Source: CAD feature listing. Evaluate the final solid. Frame: model axes, mm. A direction names the side the tool comes from. Give positions to 0.01 mm unless a question says otherwise; leave off trailing zeros. Write each loop counter-clockwise with the first axis right and the second up, starting at its lowest first coordinate (ties: lowest second). Pieces come first, ordered by that corner, then holes. Notation, with made-up numbers: (58.25, 71) - (64.25, 71) arc R27 ccw to (64.25, 89) - close; hole circle Ø7 at (49.5, 87.5). An arc over 180 degrees is marked (long way). Answer as a JSON object with one key per item and string values. Group by question number.
Autodesk Inventor part; units mm, degrees
ref_plane "YZ Plane" through (0, 0, 0) normal (1, 0, 0) x (0, 1, 0)
ref_plane "XZ Plane" through (0, 0, 0) normal (0, 1, 0) x (-1, 0, 0)
ref_plane "XY Plane" through (0, 0, 0) normal (0, 0, 1) x (1, 0, 0)
sketch "Sketch1" plane through (0, 0, 0) normal (0, 0, 1) x (1, 0, 0)
  line L0 (0, 0) -> (-75, 0)
  line L1 (-75, 0) -> (-75, 180)
  line L2 (-75, 180) -> (0, 180)
  line L3 (0, 180) -> (0, 0)
  line L4 (-65, 170) -> (-10, 170)
  line L5 (-10, 10) -> (-65, 10)
  line L6 (-65, 10) -> (-65, 85)
  line L7 (-65, 95) -> (-65, 170)
  line L8 (-10, 170) -> (-10, 95)
  line L9 (-10, 85) -> (-10, 10)
  line L10 (-65, 85) -> (-65, 95)
  line L11 (-10, 95) -> (-10, 85)
  point P0 (-65, 90)
  point P1 (-10, 90)
  dimension "d35" = 75
  dimension "d36" = 180
  dimension "d37" = 55
  dimension "d38" = 160
extrude "Extrusion7" add sketch "Sketch1" along normal blind 70
sketch "Sketch4" plane through (0, 0, 70) normal (0, 0, 1) x (1, 0, 0)
  line L0 (-75, 0) -> (0, 0)
  line L1 (0, 180) -> (-75, 180)
  line L2 (0, 0) -> (-75, 0)
  line L3 (-75, 0) -> (-75, 180)
  line L4 (-75, 180) -> (0, 180)
  line L5 (0, 180) -> (0, 0)
extrude "Extrusion8" add sketch "Sketch4" along normal blind 5
sketch "Sketch5" plane through (0, 0, 75) normal (0, 0, 1) x (1, 0, 0)
  line L0 (-65, 85) -> (-65, 95)
  line L1 (-10, 95) -> (-10, 85)
  line L2 (-10, 62.5) -> (-10, 90)
  line L3 (-10, 62.5) -> (-65, 62.5)
  line L4 (-65, 62.5) -> (-65, 117.5)
  line L5 (-65, 117.5) -> (-10, 117.5)
  line L6 (-10, 117.5) -> (-10, 62.5)
  point P0 (-65, 90)
  dimension "d59" = 55
  dimension "d60" = 55
extrude "Extrusion9" cut sketch "Sketch5" against normal blind 2
sketch "Sketch6" plane through (0, 0, 0) normal (1, 0, 0) x (0, 0, -1)
  line L0 (-10, 62.5) -> (-65, 62.5)
  line L1 (-65, 62.5) -> (-65, 117.5)
  line L2 (-65, 117.5) -> (-10, 117.5)
  line L3 (-10, 117.5) -> (-10, 62.5)
  dimension "d67" = 55
  dimension "d68" = 55
extrude "Extrusion10" cut sketch "Sketch6" against normal blind 2
sketch "Sketch7" plane through (-75, 0, 0) normal (-1, 0, 0) x (0, 0, 1)
  line L0 (10, 62.5) -> (65, 62.5)
  line L1 (10, 62.5) -> (65, 62.5)
  line L2 (65, 62.5) -> (65, 117.5)
  line L3 (65, 117.5) -> (10, 117.5)
  line L4 (10, 117.5) -> (10, 62.5)
  point P0 (0, 0)
  dimension "d71" = 55
  dimension "d72" = 55
extrude "Extrusion11" cut sketch "Sketch7" against normal blind 2
sketch "Sketch8" plane through (-75, 0, 0) normal (0, -1, 0) x (1, 0, 0)
  line L0 (10, 10) -> (65, 10)
  line L1 (65, 10) -> (65, 65)
  line L2 (65, 65) -> (10, 65)
  line L3 (10, 65) -> (10, 10)
  point P0 (75, 0)
  dimension "d75" = 55
  dimension "d76" = 55
extrude "Extrusion12" cut sketch "Sketch8" against normal blind 2
sketch "Sketch9" plane through (-75, 180, 0) normal (0, 1, 0) x (1, 0, 0)
  line L0 (10, -10) -> (65, -10)
  line L1 (65, -10) -> (65, -65)
  line L2 (65, -65) -> (10, -65)
  line L3 (10, -65) -> (10, -10)
  point P0 (75, 0)
  dimension "d79" = 55
  dimension "d80" = 55
extrude "Extrusion13" cut sketch "Sketch9" against normal blind 2
sketch "Sketch10" plane through (-75, 0, 0) normal (0, -1, 0) x (1, 0, 0)
  line L0 (74, 1) -> (63.4, 1)
  line L1 (63.4, 1) -> (63.4, 6.6)
  line L2 (63.4, 6.6) -> (74, 6.6)
  line L3 (74, 6.6) -> (74, 1)
  line L4 (1, 1) -> (11.6, 1)
  line L5 (11.6, 1) -> (11.6, 6.6)
  line L6 (11.6, 6.6) -> (1, 6.6)
  line L7 (1, 6.6) -> (1, 1)
  point P0 (75, 0)
  dimension "d83" = 10.6
  dimension "d84" = 5.6
  dimension "d85" = 10.6
  dimension "d86" = 5.6
extrude "Extrusion14" cut sketch "Sketch10" against normal blind 5
sketch "Sketch11" plane through (-75, 180, 0) normal (0, 1, 0) x (1, 0, 0)
  line L0 (1, -1) -> (11.6, -1)
  line L1 (11.6, -1) -> (11.6, -6.6)
  line L2 (11.6, -6.6) -> (1, -6.6)
  line L3 (1, -6.6) -> (1, -1)
  line L4 (74, -1) -> (63.4, -1)
  line L5 (63.4, -1) -> (63.4, -6.6)
  line L6 (63.4, -6.6) -> (74, -6.6)
  line L7 (74, -6.6) -> (74, -1)
  point P0 (75, 0)
  dimension "d89" = 10.6
  dimension "d90" = 5.6
  dimension "d91" = 10.6
  dimension "d92" = 5.6
extrude "Extrusion15" cut sketch "Sketch11" against normal blind 5
properties part number "Shoulder_Cube_TestFit_V1"
Q1. Draft query along X for faces 5 (the flat face through (0, 91, 4)), 6 (the flat face through (-75, 89, 4)), 7 (the flat face through (-38, 180, 70)), 8 (the flat face through (-69, 178, 1)). Return one class per face: released by +X, released by -X, zero draft, split by the parting line, or undercut.
Q2. First-contact query: pin 1 Ø1.5 at (x, z) = (-25.5, 39.5) entering from +Y; pin 2 Ø2 at (x, z) = (-45, 34.5) entering from -Y; pin 3 Ø12 at (y, z) = (110, 55.5) entering from -X. Flat tips, straight axial feed; report the tip coordinate or a pass-through.
Q3. Section A-A on z = 53. Return the cut outline in (x, y), then the cut area to 3 significant figures.
Q4. Ray query, probe 1 along X at (y, z) = (72.5, 26.5); probe 2 along X at (y, z) = (75, 8); probe 3 along Y at (x, z) = (-19.5, 31.5). Return the intervals inside material, ascending. Write a range as [from, to].
Q5. Reachability of faces 1 (the flat face through (-5, 91, 75)), 2 (the flat face through (-69, 2, 6.6)), 3 (the flat face through (-69, 175, 4)), 4 (the flat face through (-38, 91, 70)) from +Z, -Z, +X, -X, +Y, -Y: full face, straight path, thin tool, end or side. Return the list, or none.
Q6. Section C-C on x = -49.5. Return the cut outline in (y, z).
Q7. Section D-D on y = 106. Return the cut outline in (x, z), then the cut area to 4 significant figures.
Q8. Section B-B on y = 132.5. Return the cut outline in (x, z), then the cut area to 4 significant figures.
Taken from the geometry:
{
 "1": {"face 5": "released by +X", "face 6": "released by -X", "face 7": "zero draft", "face 8": "undercut"},
 "2": {"pin 1": "stops at y = 178", "pin 2": "stops at y = 2", "pin 3": "stops at x = -73"},
 "3": {"outline": "(-75, 0) - (-65, 0) - (-65, 2) - (-10, 2) - (-10, 0) - (0, 0) - (0, 62.5) - (-2, 62.5) - (-2, 117.5) - (0, 117.5) - (0, 180) - (-10, 180) - (-10, 178) - (-65, 178) - (-65, 180) - (-75, 180) - (-75, 117.5) - (-73, 117.5) - (-73, 62.5) - (-75, 62.5) - close; hole (-65, 10) - (-10, 10) - (-10, 170) - (-65, 170) - close", "area": "4,260 mm²"},
 "4": {"probe 1": "x = [-73, -65], [-10, -2]", "probe 2": "x = [-75, -65], [-10, 0]", "probe 3": "y = [2, 10], [170, 178]"},
 "5": {"face 1": "+Z, +X, -X, +Y, -Y", "face 2": "-Y", "face 3": "+Y", "face 4": "-Z"},
 "6": {"outline": "(0, 0) - (10, 0) - (10, 70) - (170, 70) - (170, 0) - (180, 0) - (180, 10) - (178, 10) - (178, 65) - (180, 65) - (180, 75) - (117.5, 75) - (117.5, 73) - (62.5, 73) - (62.5, 75) - (0, 75) - (0, 65) - (2, 65) - (2, 10) - (0, 10) - close"},
 "7": {"outline": "(-75, 0) - (-65, 0) - (-65, 70) - (-10, 70) - (-10, 0) - (0, 0) - (0, 10) - (-2, 10) - (-2, 65) - (0, 65) - (0, 75) - (-10, 75) - (-10, 73) - (-65, 73) - (-65, 75) - (-75, 75) - (-75, 65) - (-73, 65) - (-73, 10) - (-75, 10) - close", "area": "1,445 mm²"},
 "8": {"outline": "(-75, 0) - (-65, 0) - (-65, 70) - (-10, 70) - (-10, 0) - (0, 0) - (0, 75) - (-75, 75) - close", "area": "1,775 mm²"}
}
